For this review, take the finished solid that the model builds, in its own axes (mm). A direction names the side the tool comes from. Round coordinates to 2 decimals unless told otherwise and drop trailing zeros. Order: outer loops, then holes, each group sorted by start corner. A loop starts at its lowest first (then second) coordinate and runs counter-clockwise, first axis right, second up.
```python
from build123d import *

# Parameters (mm, degrees)
BOSS_EXTRUDE1_DEPTH = 8
SKETCH1_3_R         = 2.375
BOSS_EXTRUDE2_DEPTH = 3


with BuildPart() as part:
    # Sketch1 → Boss-Extrude1 (new body)
    with BuildSketch(Plane(origin=(0, 0, 0), x_dir=(0, 0, -1), z_dir=(1, 0, 0))):
        with BuildLine():
            ThreePointArc((-6.84422965, -1.147735338), (0.037477219, 6.939695337), (6.831434318, -1.221589567))
            Line((6.831434318, -1.221589567), (4.569647847, -24.443075278))
            Line((4.569647847, -24.443075278), (-5.036656509, -24.443075278))
            Line((-5.036656509, -24.443075278), (-6.84422965, -1.147735338))
        make_face()
        with BuildLine():
            Line((-3.768912351, -1.147735338), (-2.162031314, -21.856629017))
            Line((-2.162031314, -21.856629017), (1.73576113, -21.856629017))
            Line((1.73576113, -21.856629017), (3.745626202, -1.221589567))
            ThreePointArc((3.745626202, -1.221589567), (0.038719155, 3.939606268), (-3.768912351, -1.147735338))
        make_face(mode=Mode.SUBTRACT)
    extrude(amount=BOSS_EXTRUDE1_DEPTH)

    # Sketch1_3 → Boss-Extrude2 (add)
    with BuildSketch(Plane(origin=(0, 0, 0), x_dir=(0, 0, -1), z_dir=(1, 0, 0))):
        with BuildLine():
            ThreePointArc((-3.768912351, -1.147735338), (0.038719155, 3.939606268), (3.745626202, -1.221589567))
            Line((3.745626202, -1.221589567), (1.73576113, -21.856629017))
            Line((1.73576113, -21.856629017), (-2.162031314, -21.856629017))
            Line((-2.162031314, -21.856629017), (-3.768912351, -1.147735338))
        make_face()
        Circle(SKETCH1_3_R, mode=Mode.SUBTRACT)
    extrude(amount=BOSS_EXTRUDE2_DEPTH)


solid = part.part
```
Q1. Clearance check with flat-ended pins moving along their axes: pin 1 (2 mm diameter, centred on x = 3.5, z = -4, fed in from +Y); pin 2 (2 mm diameter, centred on x = 7, z = -2.5, fed in from +Y); pin 3 (6.5 mm diameter, centred on y = 0, z = 0, fed in from +X). State where each tip first meets the part, or that it passes through.
Q2. Take a section at C-C, the plane z = 0. State the section outline as (x, y) points (3 decimals).
Q3. Mouldability with a two-part tool opening along Z and no side actions: class faces 1 (the face through (3.944, -12.958, 5.928)), 2 (the face through (5.465, -11.684, -2.727)), 3 (the face through (4, -24.443, 0)) as +Z half, -Z half, draft (parallel to the pull), parting line (faces both ways), or undercut.
Q4. Take a section at A-A, the plane y = 0. State the section outline as (x, z) points (3 decimals).
Q5. Take a section at B-B, the plane x = 5.5. State the section outline as (y, z) points, plus the area to 3 significant figures.
Q6. Take a section at D-D, the plane x = 0.75. State the section outline as (y, z) points (3 decimals), plus the area to 3 significant figures.
Q7. Wall thickness on line 1 (Z direction, x = 4, y = 0); line 2 (Y direction, x = 0.9, z = 0) (3 decimals); line 3 (Y direction, x = 4.95, z = 0): over which ranges is each line inside the solid? List them lowest first.
Q8. Tool access review of faces 4 (the face through (5.465, -11.357, 2.977)), 5 (the face through (3.944, -12.67, -5.716)): name each direction out of +Z, -Z, +X, -X, +Y, -Y from which nothing blocks a thin tool from reaching the whole face with its end or side.
Working result:
1. pin 1: stops at y = 6.26
1. pin 2: stops at y = 6.78
1. pin 3: stops at x = 3
2. outline: (0, -24.443) - (8, -24.443) - (8, -21.857) - (3, -21.857) - (3, -2.375) - (0, -2.375) - close; (0, 2.375) - (3, 2.375) - (3, 3.94) - (8, 3.94) - (8, 6.94) - (0, 6.94) - close
3. face 1: +Z half
3. face 2: undercut
3. face 3: draft
4. outline: (0, -6.94) - (8, -6.94) - (8, -3.94) - (3, -3.94) - (3, -2.375) - (0, -2.375) - close; (0, 2.375) - (3, 2.375) - (3, 3.94) - (8, 3.94) - (8, 6.94) - (0, 6.94) - close
5. outline: (-24.44, -4.57) - (-1.22, -6.83) arc R6.94 ccw (long way) to (-1.15, 6.84) - (-24.44, 5.04) - close; hole (-21.86, -1.74) - (-1.22, -3.75) arc R3.94 ccw (long way) to (-1.15, 3.77) - (-21.86, 2.16) - close
5. area: 211 mm2
6. outline: (-24.443, -4.57) - (-1.222, -6.831) arc R6.94 ccw (long way) to (-1.148, 6.844) - (-24.443, 5.037) - close; hole circle Ø4.75 at (0, 0)
6. area: 345 mm2
7. line 1: z = -6.94 to -3.94, 3.94 to 6.94
7. line 2: y = -24.443 to -2.375, 2.375 to 6.94
7. line 3: y = -24.44 to -21.86, 3.94 to 6.94
8. face 4: +X
8. face 5: -Z, +X, -X, -Y
